For this review, take the finished solid that the model builds, in its own axes (mm). A direction names the side the tool comes from. Round coordinates to 2 decimals unless told otherwise and drop trailing zeros. Write each loop counter-clockwise with the first axis right and the second up, starting at its lowest first coordinate (ties: lowest second). Pieces come first, ordered by that corner, then holes. Notation, with made-up numbers: (-31.5, 45.25) -> (17.5, 45.25) arc R22 ccw to (17.5, 80.25) -> close; hole circle Ø2 at (30, 66.25). An arc over 180 degrees is marked (long way). Answer in a Markdown table with one row per item.
from build123d import *

# Parameters (mm, degrees)
SKETCH_1_W             = 80
SKETCH_1_H             = 36
EXTRUDE_1_DEPTH        = 15
HOLE_WIZARD_M6_1_D     = 5
HOLE_WIZARD_M6_1_DEPTH = 8
HOLE_WIZARD_M6_1_TIP   = 1.502151548
SKETCH_4_R             = 12
CUT_EXTRUDE_1_DEPTH    = 5
SKETCH_5_R             = 5
CUT_EXTRUDE_2_DEPTH    = 15
SKETCH_6_R             = 8
CUT_EXTRUDE_3_DEPTH    = 45.988887517


with BuildPart() as part:
    # 草图1 → 凸台-拉伸1 (new body)
    with BuildSketch(Plane(origin=(0, 0, 0), x_dir=(0, 0, -1), z_dir=(1, 0, 0))):
        Rectangle(SKETCH_1_W, SKETCH_1_H)
    extrude(amount=EXTRUDE_1_DEPTH)

    # M6 螺纹孔1
    with Locations(Plane.XZ.offset(18)):
        with Locations((7.5, 30), (7.5, 10), (7.5, -10), (7.5, -30)):
            Hole(HOLE_WIZARD_M6_1_D / 2, depth=HOLE_WIZARD_M6_1_DEPTH)
            with Locations((0, 0, -(HOLE_WIZARD_M6_1_DEPTH + HOLE_WIZARD_M6_1_TIP / 2))):  # 118° drill point
                Cone(0, HOLE_WIZARD_M6_1_D / 2, HOLE_WIZARD_M6_1_TIP, mode=Mode.SUBTRACT)

    # 草图4 → 切除-拉伸1 (cut)
    with BuildSketch(Plane.ZY):
        with Locations((0, 2)):
            Circle(SKETCH_4_R)
    extrude(amount=-CUT_EXTRUDE_1_DEPTH, mode=Mode.SUBTRACT)

    # 草图5 → 切除-拉伸2 (cut)
    with BuildSketch(Plane.ZY):
        with Locations((30, 2)):
            Circle(SKETCH_5_R)
    cut_extrude_2 = extrude(amount=-CUT_EXTRUDE_2_DEPTH, mode=Mode.SUBTRACT)

    # 镜向1: 切除-拉伸2 across plane
    add(cut_extrude_2.mirror(Plane.XY), mode=Mode.SUBTRACT)

    # 草图6 → 切除-拉伸3 (cut, through all)
    with BuildSketch(Plane.ZY.offset(-5)):
        with Locations((0, 2)):
            Circle(SKETCH_6_R)
    extrude(amount=-CUT_EXTRUDE_3_DEPTH, mode=Mode.SUBTRACT)


solid = part.part
1) Consider section C-C on x = 14.25. State the section outline as (y, z) points.
Solved:
| item | result |
|---|---|
| outline | (-18, -40) -> (18, -40) -> (18, 40) -> (-18, 40) -> close; hole circle Ø16 at (2, 0); hole circle Ø10 at (2, -30); hole circle Ø10 at (2, 30) |
2) Consider section D-D on y = 9. State the section outline as (x, z) points, then the cut area to 3 significant figures.
Solved:
| item | result |
|---|---|
| outline | (0, -40) -> (15, -40) -> (15, -3.87) -> (5, -3.87) -> (5, -9.75) -> (0, -9.75) -> close; (0, 9.75) -> (5, 9.75) -> (5, 3.87) -> (15, 3.87) -> (15, 40) -> (0, 40) -> close |
| area | 1,030 mm² |
3) Mouldability with a two-part tool opening along Y and no side actions: class faces 4 (the flat face through (15, -8, 1)), 5 (the cylindrical face through (2.46, 2.53, -11.99)), 6 (the conical face through (7.44, -8.76, 10.43)) as pulls with the +Y half, pulls with the -Y half, needs draft (parallel to the pull), parting line crosses it, or undercut.
Solved:
| item | result |
|---|---|
| face 4 | needs draft |
| face 5 | undercut |
| face 6 | pulls with the -Y half |
4) For line 1 (Z direction, x = 7.5, y = -14); line 2 (Y direction, x = 4.25, z = -30); line 3 (X direction, y = -14.5, z = 10), list the stretches that pass through material, from the lowest coordinate up. Write a range as [from, to].
Solved:
| item | result |
|---|---|
| line 1 | [-40, -32.5], [-27.5, -12.5], [-7.5, 7.5], [12.5, 27.5], [32.5, 40] |
| line 2 | [-18, -3], [7, 18] |
| line 3 | [0, 5], [10, 15] |
5) Consider section B-B on z = 0. State the section outline as (x, y) points, then the cut area to 3 significant figures.
Solved:
| item | result |
|---|---|
| outline | (0, -18) -> (15, -18) -> (15, -6) -> (5, -6) -> (5, -10) -> (0, -10) -> close; (0, 14) -> (5, 14) -> (5, 10) -> (15, 10) -> (15, 18) -> (0, 18) -> close |
| area | 260 mm² |
6) Consider section A-A on y = 2. State the section outline as (x, z) points.
Solved:
| item | result |
|---|---|
| outline | (0, -40) -> (15, -40) -> (15, -35) -> (0, -35) -> close; (0, -25) -> (15, -25) -> (15, -8) -> (5, -8) -> (5, -12) -> (0, -12) -> close; (0, 12) -> (5, 12) -> (5, 8) -> (15, 8) -> (15, 25) -> (0, 25) -> close; (0, 35) -> (15, 35) -> (15, 40) -> (0, 40) -> close |
7) Clearance check with a flat-ended pin moving along its axis: pin 1 Ø4.5 at (x, z) = (7.5, 10) entering from -Y. State where the tip first meets the part, or that it passes through.
Solved:
| item | result |
|---|---|
| pin 1 | y = -9.85 |
8) For faces 1 (the flat face through (7, 0, 40)), 2 (the flat face through (5, -6, 2)), 3 (the cylindrical face through (7.83, -13.94, -27.52)), list the 3-axis set-ups (+Z, -Z, +X, -X, +Y, -Y) from which the entire face can be reached by the end or side of a thin tool; tool diameter is ignored.
Solved:
| item | result |
|---|---|
| face 1 | +Z, +X, -X, +Y, -Y |
| face 2 | -X |
| face 3 | -Y |
